from build123d import *

# Parameters (mm, degrees)
SWEEP_1_PROFILE_R = 0.075


with BuildPart() as part:
    # 草图1 → 旋转1 (revolve)
    with BuildSketch(Plane(origin=(0, 0, 0), x_dir=(1, 0, 0), z_dir=(0, 1, 0))):
        Polygon((0.9, -1.75), (1.1, -1.75), (1.1, -3), (0, -3), (0, 3), (1.1, 3), (1.1, 1.75), (0.9, 1.75), align=None)
    revolve(axis=Axis((0, 0, 3), (0, 0, -1)))

    # 扫描1: sweep along a path in 草图6
    with BuildLine(Plane(origin=(0, 0, 0), x_dir=(1, 0, 0), z_dir=(0, 1, 0))) as sweep_1_path:
        Line((4.948876204, 4.25), (1.25, 4.25))
        ThreePointArc((1.25, 4.25), (0.366116524, 3.883883476), (0, 3))
    # 扫描1 profile (on start of the path) → 扫描1 (sweep)
    with BuildSketch(Plane(origin=(4.948876204, 0, -4.25), x_dir=(0, 0, -1), z_dir=(-1, 0, 0))):
        Circle(SWEEP_1_PROFILE_R)
    sweep_1 = sweep(path=sweep_1_path.line)

    # 镜向1: 扫描1 across plane
    add(sweep_1.mirror(Plane.XY))


solid = part.part
Can you work these out from the model? Positions are in its coordinate system, mm. Coordinates: 2 decimals unless noted, no trailing zeros. Loops run counter-clockwise (first coordinate to the right, second up) from the corner with the lowest first, then second, coordinate; pieces in that order, holes last. Notation, with made-up numbers: M -15,14 L 36,14 A8 cw 36,29 Z; hole C 67.5,37 d3. An arc over 180 degrees is marked long. Answer as CSV lines item,"result". Start each with the question number.
1. Suppose I cut it at A-A, the plane x = 3.25. List the corners of the cut face in (y, z) for me (3 decimals).
2. If I drill on probe 1 along Z at (x, y) = (0, 0.3); probe 2 along X at (y, z) = (-0.2, 0.75); probe 3 along X at (y, z) = (-0.35, 1), over which ranges is the centre line in solid material (lowest first)? Write a range as [from, to].
3. For pin 1 Ø0.7 at (x, y) = (0, -0.5) entering from +Z; pin 2 Ø2 at (x, z) = (1, 1) entering from +Y; pin 3 Ø0.7 at (x, y) = (0.5, 0) entering from +Z, each with a flat end and sliding along its axis, tell me the tip position at first contact or that it passes through.
4. Suppose I cut it at C-C, the plane y = -0.75. List the corners of the cut face in (x, z) for me, plus the area to 3 significant figures.
5. Suppose I cut it at D-D, the plane z = -2.5. List the corners of the cut face in (x, y) for me.
6. Suppose I cut it at B-B, the plane z = 1. List the corners of the cut face in (x, y) for me.
Output:
1,outline,"C 0,-4.25 d0.15; C 0,4.25 d0.15"
2,probe 1,"z = [-3, 3]"
2,probe 2,"x = [-0.88, 0.88]"
2,probe 3,"x = [-0.83, 0.83]"
3,pin 1,"stops at z = 3"
3,pin 2,"stops at y = 1.05"
3,pin 3,"stops at z = 4.26"
4,outline,"M -0.8,-3 L 0.8,-3 L 0.8,-1.75 L 0.5,-1.75 L 0.5,1.75 L 0.8,1.75 L 0.8,3 L -0.8,3 L -0.8,1.75 L -0.5,1.75 L -0.5,-1.75 L -0.8,-1.75 Z"
4,area,"7.51 mm^2"
5,outline,"C 0,0 d2.2"
6,outline,"C 0,0 d1.8"
